Input: part model. Units: mm. Frame: model coordinates. A direction names the side the tool comes from. Round coordinates to 2 decimals unless told otherwise and drop trailing zeros. Loops run counter-clockwise (first coordinate to the right, second up) from the corner with the lowest first, then second, coordinate; pieces in that order, holes last.
(1) Cut plane D-D, the plane z = 16. Output: boundary loops of the cut face in (x, y), and give its area (3 significant figures).
(2) Cut plane A-A, the plane z = 6.5. Output: boundary loops of the cut face in (x, y).
(3) Cut plane C-C, the plane z = 29. Output: boundary loops of the cut face in (x, y).
(4) First-contact query: pin 1 Ø2 at (x, y) = (64.5, -3) entering from -Z; pin 2 Ø4 at (x, z) = (29, 40) entering from +Y; pin 3 Ø19.5 at (y, z) = (-14, 10) entering from +X. Flat tips, straight axial feed; report the tip coordinate or a pass-through.
(5) Access query for faces 1 (the face through (60.3, -11, 10)), 2 (the face through (-56.3, -2, 5)), 3 (the face through (65, -2, 0)), 4 (the face through (-1, -2, 0)). Directions: +Z, -Z, +X, -X, +Y, -Y. A direction counts if a zero-diameter tool reaches every point of the face in a straight line with its end or side. Return the directions, or none.
(6) Cut plane B-B, the plane x = -28. Output: boundary loops of the cut face in (y, z), and give its area (3 significant figures).
(7) Line query: line 1 (X direction, y = -3, z = 3.5); line 2 (Y direction, x = -53.5, z = 56.5); line 3 (X direction, y = 6, z = 4). Output: solid intervals per line, ascending.
from build123d import *

# Parameters (mm, degrees)
F1_DEPTH = 4
F3_DEPTH = 4


with BuildPart() as f1:
    # F0 (on Front) → F1 (new body)
    with BuildSketch(Plane.XZ):
        with BuildLine():
            Line((60, 90), (-60, 90))
            ThreePointArc((-60, 90), (-67.0710678119, 87.0710678119), (-70, 80))
            Line((-70, 80), (-70, 0))
            Line((-70, 0), (-60, 0))
            Line((-60, 0), (-60, 10))
            Line((-60, 10), (-56.3, 10))
            Line((-56.3, 10), (-56.3, 0))
            Line((-56.3, 0), (56.3, 0))
            Line((56.3, 0), (56.3, 10))
            Line((56.3, 10), (60, 10))
            Line((60, 10), (60, 0))
            Line((60, 0), (70, 0))
            Line((70, 0), (70, 80))
            ThreePointArc((70, 80), (67.0710678119, 87.0710678119), (60, 90))
        make_face()
    extrude(amount=F1_DEPTH)

    # F2 (on face) → F3 (join)
    with BuildSketch(Plane.YZ.offset(56.3)):
        with BuildLine():
            Line((0, 25), (0, 10))
            Line((0, 10), (-4, 10))
            Line((-4, 10), (-4, 25))
            ThreePointArc((-4, 25), (-4.9283988219, 24.7714614383), (-5.6446227124, 24.1380756275))
            Line((-5.6446227124, 24.1380756275), (-21.8974136828, 0.6513155869))
            Line((-21.8974136828, 0.6513155869), (14.6343906331, -0.67813536))
            Line((14.6343906331, -0.67813536), (1.7724384249, 23.9265322606))
            ThreePointArc((1.7724384249, 23.9265322606), (1.0360828825, 24.7107110395), (0, 25))
        make_face()
    extrude(amount=F3_DEPTH)


solid = f1.part
Reported:
1. outline: (-70, -4) - (56.3, -4) - (56.3, -11.28) - (60.3, -11.28) - (60.3, -4) - (70, -4) - (70, 0) - (60.3, 0) - (60.3, 5.92) - (56.3, 5.92) - (56.3, 0) - (-70, 0) - close
1. area: 613 mm2
2. outline: (-70, -4) - (-60, -4) - (-60, 0) - (-70, 0) - close; (-56.3, -4) - (56.3, -4) - (56.3, -17.85) - (60.3, -17.85) - (60.3, -4) - (70, -4) - (70, 0) - (60.3, 0) - (60.3, 10.88) - (56.3, 10.88) - (56.3, 0) - (-56.3, 0) - close
3. outline: (-70, -4) - (70, -4) - (70, 0) - (-70, 0) - close
4. pin 1: stops at z = 0
4. pin 2: stops at y = 0
4. pin 3: stops at x = 60.3
5. face 1: +Z, -Z, +X, -Y
5. face 2: -Z, +Y, -Y
5. face 3: -Z, +X, +Y, -Y
5. face 4: -Z, -X, +Y, -Y
6. outline: (-4, 0) - (0, 0) - (0, 90) - (-4, 90) - close
6. area: 360 mm2
7. line 1: x = -70 to -60, -56.3 to 70
7. line 2: y = -4 to 0
7. line 3: x = 56.3 to 60.3
